Could you check a few things on this model? Use its own coordinates, in mm. Coordinates: 2 decimals unless noted, no trailing zeros. Order: outer loops, then holes, each group sorted by start corner. A loop starts at its lowest first (then second) coordinate and runs counter-clockwise, first axis right, second up. Notation, with made-up numbers: (44, -7.5) - (64, -7.5) arc R19 cw to (64, 28.5) - close; hole circle Ø4 at (35, 0). An arc over 180 degrees is marked (long way). One line per item, written item: value.
from build123d import *

# Parameters (mm, degrees)
SKETCH1_W           = 427
SKETCH1_H           = 35
BOSS_EXTRUDE1_DEPTH = 4
SKETCH2_R           = 11.9
SKETCH2_R_2         = 1.6
SKETCH2_R_3         = 5.7
SKETCH2_R_4         = 1.7
CUT_EXTRUDE1_DEPTH  = 4


with BuildPart() as part:
    # Sketch1 → Boss-Extrude1 (new body)
    with BuildSketch(Plane.XY):
        Rectangle(SKETCH1_W, SKETCH1_H)
    extrude(amount=BOSS_EXTRUDE1_DEPTH)

    # Sketch2 → Cut-Extrude1 (cut)
    with BuildSketch(Plane.XY.offset(4)):
        with Locations((-20.271803936, 2)):
            Circle(SKETCH2_R)
        with Locations((-30.271803936, -9.5)):
            Circle(SKETCH2_R_2)
        with Locations((-10.271803936, 13.5)):
            Circle(SKETCH2_R_2)
        with Locations((-58.211803936, -9.5)):
            Circle(SKETCH2_R_2)
        with Locations((-48.211803936, 2)):
            Circle(SKETCH2_R)
        with Locations((-38.211803936, 13.5)):
            Circle(SKETCH2_R_2)
        with Locations((126.64, -11.5)):
            Circle(SKETCH2_R_2)
        with Locations((146.64, 11.5)):
            Circle(SKETCH2_R_2)
        with Locations((136.64, 0)):
            Circle(SKETCH2_R)
        with Locations((166.76, -11.5)):
            Circle(SKETCH2_R_2)
        with Locations((186.76, 11.5)):
            Circle(SKETCH2_R_2)
        with Locations((176.76, 0)):
            Circle(SKETCH2_R)
        with Locations((-104.091803936, -4.865)):
            Circle(SKETCH2_R_3)
        with Locations((86.52, -9.5)):
            Circle(SKETCH2_R_2)
        with Locations((106.52, 13.5)):
            Circle(SKETCH2_R_2)
        with Locations((68.58, 2)):
            Circle(SKETCH2_R)
        with Locations((96.52, 2)):
            Circle(SKETCH2_R)
        with Locations((12.7, -4.865)):
            Circle(SKETCH2_R_3)
        with Locations((78.58, 13.5)):
            Circle(SKETCH2_R_2)
        with Locations((58.58, -9.5)):
            Circle(SKETCH2_R_2)
        with Locations((-127.5, 0)):
            Circle(SKETCH2_R_4)
        with Locations((-183.5, 0)):
            Circle(SKETCH2_R_4)
        with BuildLine():
            Line((-178.05, -14.05), (-132.95, -14.05))
            ThreePointArc((-132.95, -14.05), (-132.242893219, -13.757106781), (-131.95, -13.05))
            Line((-131.95, -13.05), (-131.95, 13.05))
            ThreePointArc((-131.95, 13.05), (-132.242893219, 13.757106781), (-132.95, 14.05))
            Line((-132.95, 14.05), (-178.05, 14.05))
            ThreePointArc((-178.05, 14.05), (-178.757106781, 13.757106781), (-179.05, 13.05))
            Line((-179.05, 13.05), (-179.05, -13.05))
            ThreePointArc((-179.05, -13.05), (-178.757106781, -13.757106781), (-178.05, -14.05))
        make_face()
    extrude(amount=-CUT_EXTRUDE1_DEPTH, mode=Mode.SUBTRACT)


solid = part.part
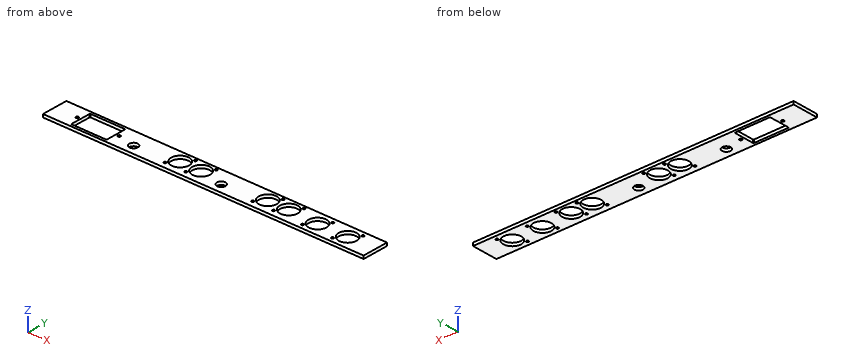
Item 1: If I drill on probe 1 along Y at (x, z) = (-138, 2.25); probe 2 along Y at (x, z) = (-183.5, 2); probe 3 along Y at (x, z) = (186.5, 0.95), over which ranges is the centre line in solid material (lowest first)?
Conclusion:
probe 1: -17.5 to -14.05, 14.05 to 17.5
probe 2: -17.5 to -1.7, 1.7 to 17.5
probe 3: -17.5 to -6.84, 6.84 to 9.92, 13.08 to 17.5
Item 2: I want a section at B-B on z = 0.75. Give the number of separate pieces and of enclosed holes in the cut face, then the cut area to 3 significant figures.
Conclusion:
separate pieces: 1
enclosed holes: 23
area: 10,600 mm²
Item 3: I want a section at A-A on x = 12.7. Please give me the cut outline in (y, z) (3 decimals), then the cut area to 3 significant figures.
Conclusion:
outline: (-17.5, 0) - (-10.565, 0) - (-10.565, 4) - (-17.5, 4) - close; (0.835, 0) - (17.5, 0) - (17.5, 4) - (0.835, 4) - close
area: 94.4 mm²
Item 4: I'm going to push a flat-ended pin straight in: pin 1 Ø3 at (x, y) = (-127.5, 0) entering from -Z (3 decimals). Where does the tip first touch, or does it pass through?
Conclusion:
pin 1: through
Item 5: I want a section at C-C on x = -167. Please give me the cut outline in (y, z), then the cut area to 3 significant figures.
Conclusion:
outline: (-17.5, 0) - (-14.05, 0) - (-14.05, 4) - (-17.5, 4) - close; (14.05, 0) - (17.5, 0) - (17.5, 4) - (14.05, 4) - close
area: 27.6 mm²
